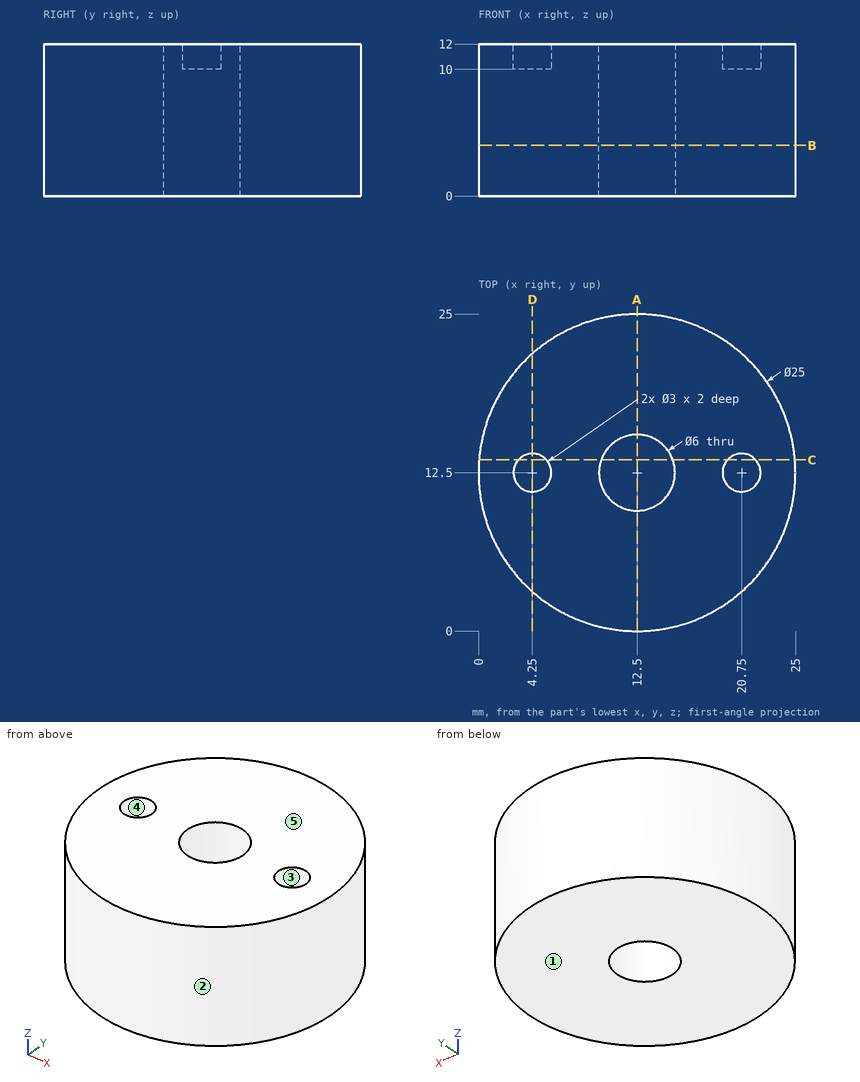
Source: three-view drawing plus pictorial views. Frame: mm from the lowest corner of the part. A direction names the side the tool comes from. Coordinates: 2 decimals unless noted, no trailing zeros. Loops run counter-clockwise (first coordinate to the right, second up) from the corner with the lowest first, then second, coordinate; pieces in that order, holes last. Notation, with made-up numbers: M 79.5,58.5 L 108.5,58.5 A32 cw 108.5,93.5 Z; hole C 50.25,18 d6. An arc over 180 degrees is marked long. Use CSV: the item, a comma, the result in double quotes.
(1) Reachability of the marked faces 4 and 5 from +Z, -Z, +X, -X, +Y, -Y: full face, straight path, thin tool, end or side. Return the list, or none.
Answers follow:
face 4,"+Z"
face 5,"+Z, +X, -X, +Y, -Y"
(2) Cut plane B-B on z = 4. Return loops of the section in (x, y), and give its area (3 significant figures).
Answers follow:
outline,"C 12.5,12.5 d25; hole C 12.5,12.5 d6"
area,"463 mm²"
(3) Contact query for flat-ended pins moving along their axis: pin 1 (6 mm diameter, centred on x = 22, z = 10.5, fed in from +Y); pin 2 (3 mm diameter, centred on x = 14.5, z = 5, fed in from +Y); pin 3 (4 mm diameter, centred on y = 9.5, z = 10, fed in from -X). Output: stop coordinate, or through.
Answers follow:
pin 1,"y = 23.18"
pin 2,"y = 24.99"
pin 3,"x = 0.04"
(4) Line query: line 1 (Y direction, x = 12.5, z = 5); line 2 (Y direction, x = 4.25, z = 10.6); line 3 (X direction, y = 10.5, z = 3.5). Output: solid intervals per line, ascending. Write a range as [from, to].
Answers follow:
line 1,"[0, 9.5], [15.5, 25]"
line 2,"[3.11, 11], [14, 21.89]"
line 3,"[0.16, 10.26], [14.74, 24.84]"
(5) Cut plane A-A on x = 12.5. Return loops of the section in (y, z).
Answers follow:
outline,"M 0,0 L 9.5,0 L 9.5,12 L 0,12 Z; M 15.5,0 L 25,0 L 25,12 L 15.5,12 Z"
(6) Cut plane D-D on x = 4.25. Return loops of the section in (y, z), and give its area (3 significant figures).
Answers follow:
outline,"M 3.11,0 L 21.89,0 L 21.89,12 L 14,12 L 14,10 L 11,10 L 11,12 L 3.11,12 Z"
area,"219 mm²"
(7) Cut plane C-C on y = 13.5. Return loops of the section in (x, z), and give its area (3 significant figures).
Answers follow:
outline,"M 0.04,0 L 9.67,0 L 9.67,12 L 5.37,12 L 5.37,10 L 3.13,10 L 3.13,12 L 0.04,12 Z; M 15.33,0 L 24.96,0 L 24.96,12 L 21.87,12 L 21.87,10 L 19.63,10 L 19.63,12 L 15.33,12 Z"
area,"222 mm²"
(8) Draft query along Y for the marked faces 1, 2 and 3. Return one class per face: pulls with the +Y half, pulls with the -Y half, needs draft (parallel to the pull), parting line crosses it, or undercut.
Answers follow:
face 1,"needs draft"
face 2,"parting line crosses it"
face 3,"undercut"
